```python
from build123d import *

# Parameters (mm, degrees)
SKETCH1_R           = 20
BOSS_EXTRUDE1_DEPTH = 10
SKETCH3_R           = 2.5
CUT_EXTRUDE1_DEPTH  = 5
SKETCH4_R           = 2.5
BOSS_EXTRUDE2_DEPTH = 2


with BuildPart() as part:
    # Sketch1 → Boss-Extrude1 (new body)
    with BuildSketch(Plane(origin=(0, 0, 0), x_dir=(1, 0, 0), z_dir=(0, 1, 0))):
        Circle(SKETCH1_R)
    extrude(amount=BOSS_EXTRUDE1_DEPTH)

    # Sketch2 → Revolve1 (revolve)
    with BuildSketch(Plane(origin=(0, 0, 0), x_dir=(0, 0, -1), z_dir=(1, 0, 0))):
        with BuildLine():
            Line((20, 10), (25, 10))
            Line((25, 10), (25, 7.5))
            Line((25, 7.5), (20.872288151, 6.191567774))
            ThreePointArc((20.872288151, 6.191567774), (20, 5), (20.872288151, 3.808432226))
            Line((20.872288151, 3.808432226), (25, 2.5))
            Line((25, 2.5), (25, 0))
            Line((25, 0), (20, 0))
            Line((20, 0), (19.25, 0))
            Line((19.25, 0), (19.25, 10))
            Line((19.25, 10), (20, 10))
        make_face()
    revolve(axis=Axis((0, 10, 0), (0, -1, 0)))

    # Sketch3 → Cut-Extrude1 (cut)
    with BuildSketch(Plane.XZ):
        Circle(SKETCH3_R)
    extrude(amount=-CUT_EXTRUDE1_DEPTH, mode=Mode.SUBTRACT)

    # Sketch4 → Boss-Extrude2 (add)
    with BuildSketch(Plane(origin=(0, 10, 0), x_dir=(1, 0, 0), z_dir=(0, 1, 0))):
        with Locations((0, -15)):
            Circle(SKETCH4_R)
    extrude(amount=BOSS_EXTRUDE2_DEPTH)


solid = part.part
```
CAD build for the part. Positions are in the model's coordinates, mm. A direction names the side the tool comes from. Round coordinates to 2 decimals unless told otherwise and drop trailing zeros. Loops run counter-clockwise (first coordinate to the right, second up) from the corner with the lowest first, then second, coordinate; pieces in that order, holes last. Notation, with made-up numbers: (58.5, 45.25) - (69.5, 45.25) arc R8 ccw to (69.5, 54.25) - close; hole circle Ø7 at (82.5, 15.5). An arc over 180 degrees is marked (long way). Return JSON: item names as keys, results as strings. Group by question number.
Q1. Band-saw the part on A-A on z = 0. Give the cut face in (x, y).
Q2. Flat gauge pins, fed straight in: pin 1 Ø15 at (x, z) = (-4, -12) entering from +Y; pin 2 Ø2.5 at (x, z) = (1, 0.5) entering from -Y; pin 3 Ø3 at (x, y) = (-6, 10) entering from +Z. Where does each tip first touch, or does it go through?
Q3. Tool access for faces 5 (the face through (-5, 0, 0)), 6 (the face through (-0.54, 2.46, -2.44)), 7 (the face through (-0.54, 10.99, 17.44)): list every direction of +Z, -Z, +X, -X, +Y, -Y with a clear straight run to the whole face (end or side of a thin tool).
Q4. Band-saw the part on B-B on x = 0. Give the cut face in (y, z).
Q5. Two-plate mould, pull along Y, no slides. Class faces 1 (the face through (7.509, 8.732, -23.846)), 2 (the face through (0, 12, 15)), 3 (the face through (-20.572, 6.255, 4.568)), 4 (the face through (-20.628, 3.727, 4.581)): +Y half, -Y half, draft (parallel to the pull), parting line (faces both ways), or undercut.
Q6. Drill centre lines: line 1 along Y through (x, z) = (6, -20); line 2 along Y through (x, z) = (7, 6); line 3 along Y through (x, z) = (4.5, 23). Where is each one in solid material? Low to high. Write a range as [from, to].
Solutions:
{
 "1": {"outline": "(-25, 0) - (-2.5, 0) - (-2.5, 5) - (2.5, 5) - (2.5, 0) - (25, 0) - (25, 2.5) - (20.87, 3.81) arc R1.25 cw to (20.87, 6.19) - (25, 7.5) - (25, 10) - (-25, 10) - (-25, 7.5) - (-20.87, 6.19) arc R1.25 cw to (-20.87, 3.81) - (-25, 2.5) - close"},
 "2": {"pin 1": "stops at y = 10", "pin 2": "stops at y = 5", "pin 3": "stops at z = 24.59"},
 "3": {"face 5": "+Z, -Z, +X, -X, -Y", "face 6": "-Y", "face 7": "+Y"},
 "4": {"outline": "(0, -25) - (2.5, -25) - (3.81, -20.87) arc R1.25 cw to (6.19, -20.87) - (7.5, -25) - (10, -25) - (10, 12.5) - (12, 12.5) - (12, 17.5) - (10, 17.5) - (10, 25) - (7.5, 25) - (6.19, 20.87) arc R1.25 cw to (3.81, 20.87) - (2.5, 25) - (0, 25) - (0, 2.5) - (5, 2.5) - (5, -2.5) - (0, -2.5) - close"},
 "5": {"face 1": "draft", "face 2": "+Y half", "face 3": "undercut", "face 4": "undercut"},
 "6": {"line 1": "y = [0, 3.81], [6.19, 10]", "line 2": "y = [0, 10]", "line 3": "y = [0, 3], [7, 10]"}
}
